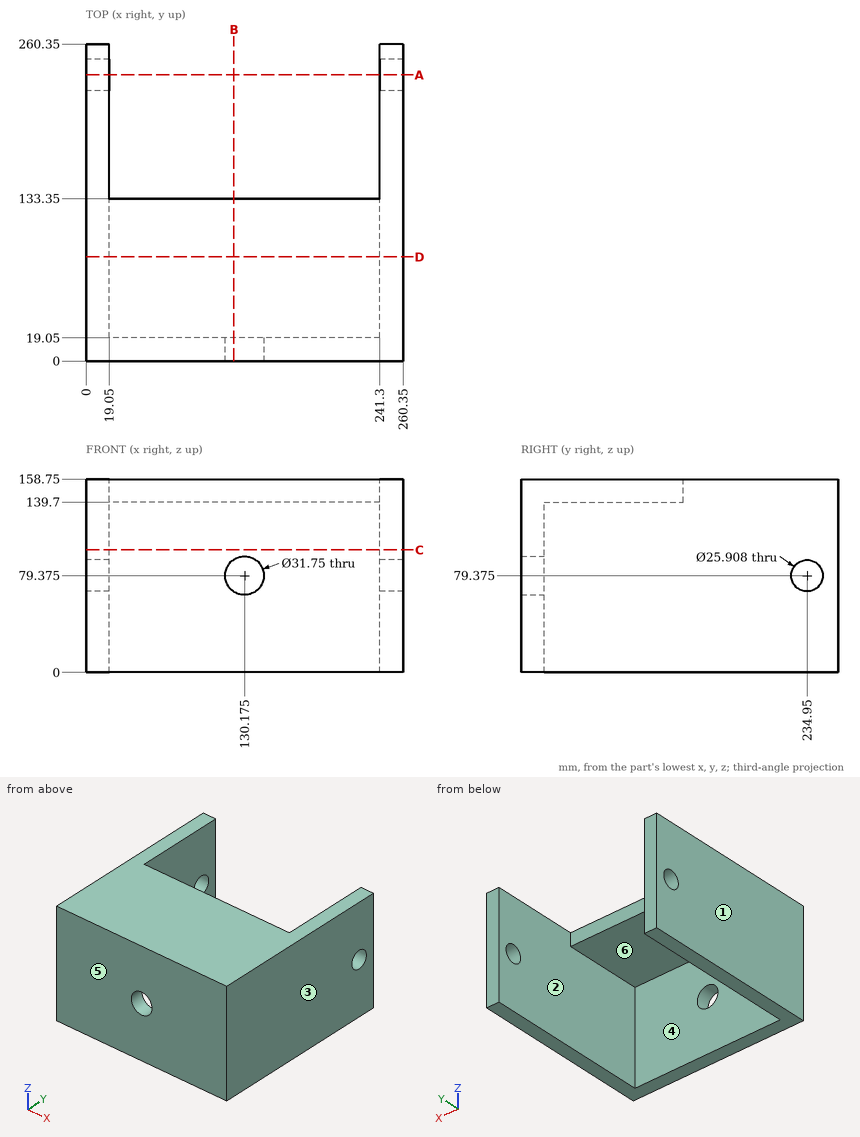
Could you check a few things on this drawing? It's one solid part, dimensions in mm from its lowest x, y, z. A direction names the side the tool comes from. Coordinates: 2 decimals unless noted, no trailing zeros. Order: outer loops, then holes, each group sorted by start corner. A loop starts at its lowest first (then second) coordinate and runs counter-clockwise, first axis right, second up. Notation, with made-up numbers: M -32.75,9 L -14.75,9 A32 ccw -14.75,42 Z; hole C -30.75,41 d6. An arc over 180 degrees is marked long. Use a Markdown table: item, result. Add a question column.
Q1. If I drill on L1, parallel to X at y = 109, z = 7.5; L2, parallel to Z at x = 10, y = 234; L3, parallel to Y at x = 197.5, z = 143.5, over which ranges is the centre line in solid material (lowest first)?
Q2. We'd pull the mould along X, two halves only. Please class the marked faces 3, 4, 5 and 6: pulls with the +X half, pulls with the -X half, needs draft (parallel to the pull), parting line crosses it, or undercut.
Q3. I want a section at C-C on z = 100.5. List the corners of the cut face in (x, y) for me, then the cut area to 3 significant figures.
Q4. I want a section at A-A on y = 234.95. List the corners of the cut face in (x, z) for me, then the cut area to 3 significant figures.
Q5. Which directions (+Z, -Z, +X, -X, +Y, -Y) give clear straight access to the entire face, cutting with the end or side of a thin tool? Please do the marked faces 1 and 2.
Q6. I want a section at B-B on x = 121.5. List the corners of the cut face in (y, z) for me, then the cut area to 3 significant figures.
Q7. I want a section at D-D on y = 85.5. List the corners of the cut face in (x, z) for me.
Q8. I'm going to push flat-ended pins straight in: pin 1 (3 mm diameter, centred on x = 62, z = 51.5, fed in from +Y); pin 2 (23.5 mm diameter, centred on y = 234.95, z = 79.375, fed in from +X); pin 3 (21 mm diameter, centred on x = 123, z = 149, fed in from +Y). Where does each tip first touch, or does it pass through?
Checked values:
| question | item | result |
|---|---|---|
| 1 | L1 | 0 to 19.05, 241.3 to 260.35 |
| 1 | L2 | 0 to 66.46, 92.29 to 158.75 |
| 1 | L3 | 0 to 133.35 |
| 2 | face 3 | pulls with the +X half |
| 2 | face 4 | undercut |
| 2 | face 5 | needs draft |
| 2 | face 6 | undercut |
| 3 | outline | M 0,0 L 260.35,0 L 260.35,260.35 L 241.3,260.35 L 241.3,19.05 L 19.05,19.05 L 19.05,260.35 L 0,260.35 Z |
| 3 | area | 14,200 mm² |
| 4 | outline | M 0,0 L 19.05,0 L 19.05,66.42 L 0,66.42 Z; M 0,92.33 L 19.05,92.33 L 19.05,158.75 L 0,158.75 Z; M 241.3,0 L 260.35,0 L 260.35,66.42 L 241.3,66.42 Z; M 241.3,92.33 L 260.35,92.33 L 260.35,158.75 L 241.3,158.75 Z |
| 4 | area | 5,060 mm² |
| 5 | face 1 | +Z, -Z, -X, +Y, -Y |
| 5 | face 2 | -Z, +Y |
| 6 | outline | M 0,0 L 19.05,0 L 19.05,66.08 L 0,66.08 Z; M 0,92.67 L 19.05,92.67 L 19.05,139.7 L 133.35,139.7 L 133.35,158.75 L 0,158.75 Z |
| 6 | area | 4,700 mm² |
| 7 | outline | M 0,0 L 19.05,0 L 19.05,139.7 L 241.3,139.7 L 241.3,0 L 260.35,0 L 260.35,158.75 L 0,158.75 Z |
| 8 | pin 1 | y = 19.05 |
| 8 | pin 2 | through |
| 8 | pin 3 | y = 133.35 |
